The listing builds one solid part. Answer for the finished solid, in the listing's coordinates (mm). Face numbers are marked on the shaded views. A direction names the side the tool comes from. Coordinates: 2 decimals unless noted, no trailing zeros. Loops run counter-clockwise (first coordinate to the right, second up) from the corner with the lowest first, then second, coordinate; pieces in that order, holes last. Notation, with made-up numbers: M 69.25,77 L 109.25,77 A20 ccw 109.25,95 Z; hole C -25.5,-30.75 d3. An arc over 180 degrees is marked long. Return JSON: item names as keys, results as strings. Group by question number.
1. Given P1, Ø3, axis at y = -103.5, z = -16, coming from the -X side; P2, Ø5, axis at y = 6.5, z = -7.5, coming from the +X side; P3, Ø5, axis at x = 54.21, y = -64.5, coming from the +Z side, each flat-ended and moving along its own axis, determine where each tip first touches the part or whether it passes through.
2. The mould has two halves that part along X. Classify the marked faces 4, 5 and 6: pulls with the +X half, pulls with the -X half, needs draft (parallel to the pull), parting line crosses it, or undercut.
3. Section D-D (x = 62) is taken. Write down the section's boundary in (y, z).
4. Section B-B (x = 33) is taken. Write down the section's boundary in (y, z), then the cut area to 3 significant figures.
5. Section C-C (y = -51) is taken. Write down the section's boundary in (x, z).
6. Which of the six approach directions +Z, -Z, +X, -X, +Y, -Y give full straight-line access (tool end or side, diameter ignored) to the marked faces 1, 2 and 3?
7. Section A-A (z = 10) is taken. Write down the section's boundary in (x, y).
8. Straight lines are drawn through the part: L1, parallel to Z at x = 0, y = 7.5; L2, parallel to Y at x = 62, z = -13; L3, parallel to Y at x = 1, z = -15. For each, find the intervals that lie inside material, in ascending order. Write a range as from..to.
Autodesk Inventor part; units mm, degrees
ref_plane "YZ Plane" through (0, 0, 0) normal (1, 0, 0) x (0, 1, 0)
ref_plane "XZ Plane" through (0, 0, 0) normal (0, 1, 0) x (-1, 0, 0)
ref_plane "XY Plane" through (0, 0, 0) normal (0, 0, 1) x (1, 0, 0)
sketch "Sketch1" plane through (0, 0, 0) normal (0, 1, 0) x (-1, 0, 0)
  circle A0 centre (0, 10) radius 4
  circle A1 centre (0, -10) radius 4
  line L0 (10, 20) -> (-50, 20)
  line L1 (-50, 20) -> (-50, -20)
  line L2 (-50, -20) -> (10, -20)
  line L3 (10, -20) -> (10, 20)
  line L4 (0, 10) -> (0, -10)
  point P0 (0, 0)
  point P1 (0, 0)
  dimension "d0" = 8
  dimension "d1" = 40
  dimension "d2" = 20
  dimension "d3" = 10
extrude "Extrusion1" add sketch "Sketch1" along normal blind 10
sketch "Sketch2" plane through (50, 0, -20) normal (0, 0, -1) x (-1, 0, 0)
  circle A0 centre (-12, -60) radius 57.5 construction
  line L0 (0, 0) -> (60, 0)
  line L1 (0, 0) -> (-23.9149, -54.8004)
  line L2 (-0.0851, -65.1996) -> (28.3679, 0)
  circle A1 centre (-12, -60) radius 9 construction
  circle A2 centre (-4.2058, -64.5) radius 1.5
  circle A3 centre (-19.7942, -64.5) radius 1.5
  circle A4 centre (-12, -51) radius 1.5
  circle A5 centre (-12, -60) radius 13
  line L3 (-19.7942, -64.5) -> (-4.2058, -64.5) construction
  line L4 (-12, -51) -> (-4.2058, -64.5) construction
  line L5 (-19.7942, -64.5) -> (-12, -51) construction
  arc A6 (33.3679, 0) -> (24.0722, -9.8435) centre (42.4028, -17.843) ccw
  line L6 (0, 0) -> (0, 10)
  line L7 (-19.4144, -70.6783) -> (44, -114.7095)
  line L8 (44, -114.7095) -> (54, -114.7095)
  line L9 (54, -114.7095) -> (54, -90)
  line L10 (54, -90) -> (-4.5856, -49.3217)
  line L11 (0, 0) -> (0, 10)
  arc A7 (8.1288, -46.3777) -> (12.283, -61.0342) centre (19.1271, -51.1773) ccw
  circle A8 centre (-12, -60) radius 6
  point P0 (50, 0)
  point P1 (4.1861, -55.4122)
  dimension "d6" = 115
  dimension "d7" = 3
  dimension "d8" = 18
  dimension "d9" = 26
  dimension "d10" = 60
  dimension "d11" = 12
  dimension "d12" = 5
  dimension "d13" = 20
  dimension "d15" = 66
  dimension "d18" = 10
  dimension "d19" = 30
  dimension "d20" = 12
  dimension "d21" = 12
extrude "Extrusion2" add sketch "Sketch2" against normal blind 10
sketch "Sketch3" plane through (50, 0, -10) normal (0, 0, 1) x (1, 0, 0)
  circle A0 centre (-49, -95.3547) radius 2
  circle A1 centre (-49, -109.3547) radius 2
  line L0 (-54, -90) -> (-44, -90)
  line L1 (-44, -90) -> (-44, -114.7095)
  line L2 (-44, -114.7095) -> (-54, -114.7095)
  line L3 (-54, -114.7095) -> (-54, -90)
  line L4 (-49, -95.3547) -> (-49, -109.3547)
  point P0 (-50, 0)
  point P1 (-44, -102.3547)
  point P2 (-49, -102.3547)
  point P3 (-49, -90)
  dimension "d24" = 4
  dimension "d25" = 14
extrude "Extrusion3" cut sketch "Sketch3" against normal blind 10 contours A0 | A1
properties part number "Mount_Frame"
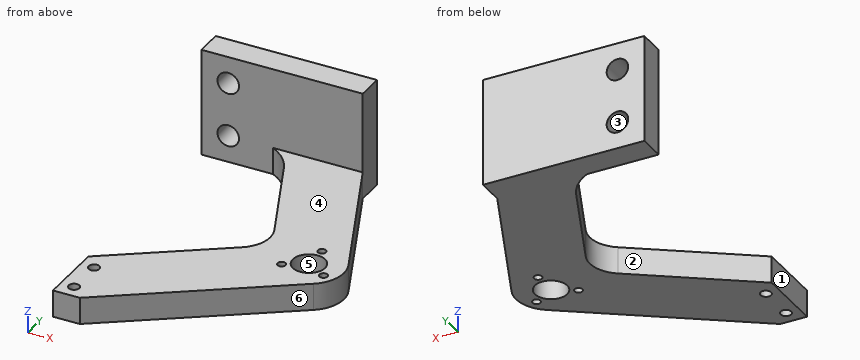
Worked out:
{
 "1": {"P1": "x = -4", "P2": "x = 50", "P3": "z = -10"},
 "2": {"face 4": "needs draft", "face 5": "undercut", "face 6": "pulls with the +X half"},
 "3": {"outline": "M -75.83,-20 L -66,-20 L -66,-10 L -75.83,-10 Z; M -54,-20 L -52.5,-20 L -52.5,-10 L -54,-10 Z; M -49.5,-20 L -27.5,-20 L -27.5,-10 L -49.5,-10 Z"},
 "4": {"outline": "M -95.96,-20 L -64.31,-20 L -64.31,-10 L -95.96,-10 Z; M -26.05,-20 L 10,-20 L 10,20 L 0,20 L 0,-10 L -26.05,-10 Z", "area": "977 mm^2"},
 "5": {"outline": "M 42.87,-20 L 60.5,-20 L 60.5,-10 L 42.87,-10 Z; M 63.5,-20 L 72.26,-20 L 72.26,-10 L 63.5,-10 Z"},
 "6": {"face 1": "+Z, -Z, -X, -Y", "face 2": "+Z, -Z, -X", "face 3": "+Y"},
 "7": {"outline": "M -10,0 L -4,0 L -4,10 L -10,10 Z; M 4,0 L 50,0 L 50,10 L 4,10 Z"},
 "8": {"L1": "-20..-14, -6..6, 14..20", "L2": "-75.83..-66, -54..-52.5, -49.5..-27.5", "L3": "-114.71..-111.35, -107.35..-97.35, -93.35..-86.53, 0..10"}
}
